Geometry check sheet. Reference: the model listing, model coordinates, mm. A direction names the side the tool comes from. Coordinates: 2 decimals unless noted, no trailing zeros. One line per question, with ' | ' between items.
from build123d import *

# Parameters (mm, degrees)
SKETCH2_W                   = 25.4
SKETCH2_H                   = 25.4
FILLET1_R                   = 3.175
SHELL1_T                    = -1.5875
SKETCH3_R                   = 3.175
WOOD_HOLE_DEPTH             = 1.5875
LPATTERN1_COUNT             = 7
LPATTERN1_PITCH             = 63.5
SKETCH5_R                   = 3.175
CONT_MTG_DEPTH              = 470.9
F_1_4_0_25_DIAMETER_HOLE1_D = 6.35
SKETCH8_R                   = 3.571875
CUT_EXTRUDE1_DEPTH          = 26.4
LPATTERN2_COUNT             = 2
LPATTERN2_PITCH             = 25.4


with BuildPart() as part:
    # Base-Sweep: sweep along a path in Sketch1
    with BuildLine(Plane.XY) as base_sweep_path:
        Line((0, 0), (406.4, 0))
        ThreePointArc((406.4, 0), (442.321024484, -14.878975516), (457.2, -50.8))
        Line((457.2, -50.8), (457.2, -914.4))
    # Sketch2 (on Right Plane) → Base-Sweep (sweep)
    with BuildSketch(Plane(origin=(0, 0, 0), x_dir=(0, 0, -1), z_dir=(1, 0, 0))):
        Rectangle(SKETCH2_W, SKETCH2_H)
    sweep(path=base_sweep_path.line)

    # Fillet1
    fillet1_edges = [part.edges().sort_by_distance(p)[0] for p in [
        (451.301280605, -5.898719395, 12.7),
        (451.301280605, -5.898719395, -12.7),
        (433.340768363, -23.859231637, -12.7),
        (433.340768363, -23.859231637, 12.7),
        (469.9, -482.6, 12.7),
        (469.9, -482.6, -12.7),
        (444.5, -482.6, -12.7),
        (444.5, -482.6, 12.7),
        (203.2, 12.7, 12.7),
        (203.2, 12.7, -12.7),
        (203.2, -12.7, -12.7),
        (203.2, -12.7, 12.7),
    ]]
    fillet(fillet1_edges, radius=FILLET1_R)

    # Shell1
    shell1_openings = [part.faces().sort_by_distance(p)[0] for p in [
        (457.2, -914.4, 0),
        (0, 0, 0),
    ]]
    offset(amount=SHELL1_T, openings=shell1_openings, kind=Kind.INTERSECTION)

    # Sketch3 → Wood Hole (cut)
    with BuildSketch(Plane(origin=(0, 12.7, 0), x_dir=(-1, 0, 0), z_dir=(0, 1, 0))):
        with Locations((-12.7, 0)):
            Circle(SKETCH3_R)
    wood_hole = extrude(amount=-WOOD_HOLE_DEPTH, mode=Mode.SUBTRACT)

    # LPattern1: Wood Hole ×7
    with Locations(*[(i * LPATTERN1_PITCH, 0, 0) for i in range(1, LPATTERN1_COUNT)]):
        add(wood_hole, mode=Mode.SUBTRACT)

    # Sketch5 → cont_mtg (cut, through all)
    with BuildSketch(Plane(origin=(469.9, 0, 0), x_dir=(0, 0, -1), z_dir=(1, 0, 0))):
        with Locations((0, -109.5375)):
            Circle(SKETCH5_R)
        with Locations((0, -134.9375)):
            Circle(SKETCH5_R)
    extrude(amount=-CONT_MTG_DEPTH, mode=Mode.SUBTRACT)

    # 1/4 (0.25) Diameter Hole1 (through all)
    with Locations(Plane.XY.offset(12.7)):
        with Locations((177.8, 0), (355.6, 0)):
            Hole(F_1_4_0_25_DIAMETER_HOLE1_D / 2)

    # Sketch8 → Cut-Extrude1 (cut, through all)
    with BuildSketch(Plane(origin=(0, 0, -12.7), x_dir=(-1, 0, 0), z_dir=(0, 0, -1))):
        with Locations((-457.2, -889)):
            Circle(SKETCH8_R)
    cut_extrude1 = extrude(amount=-CUT_EXTRUDE1_DEPTH, mode=Mode.SUBTRACT)

    # LPattern2: Cut-Extrude1 ×2
    with Locations(*[(0, i * LPATTERN2_PITCH, 0) for i in range(1, LPATTERN2_COUNT)]):
        add(cut_extrude1, mode=Mode.SUBTRACT)


solid = part.part
1. Go/stop test with flat-tipped pins: P1, Ø10, axis at y = -134.94, z = 0, coming from the -X side; P2, Ø10, axis at x = 139.7, z = 0, coming from the -Y side; P3, Ø5, axis at x = 12.7, z = 0, coming from the +Y side; P4, Ø7.5, axis at x = 177.8, y = 0, coming from the -Z side. Record where each tip stops, or that it passes through.
Worked answers:
P1: x = 444.5 | P2: y = -12.7 | P3: y = -11.11 | P4: z = -12.7
2. Material ranges on line 1 (Y direction, x = 175, z = -8); line 2 (X direction, y = -116, z = -0.25); line 3 (Y direction, x = 177.8, z = -12.2) (3 decimals), recorded low to high. Write a range as from..to.
Worked answers:
line 1: -12.7..-11.11, 11.11..12.7 | line 2: 444.5..446.09, 468.31..469.9 | line 3: -11.235..-3.175, 3.175..11.235
3. Tool access check on faces 5 (the face through (206, -11.112, 0)), 6 (the face through (468.312, -489, 0)), 7 (the face through (434.153, -22.43, -0.133)), 8 (the face through (206, -12.7, 0)), 9 (the face through (0, -1, -11.3)). Record the directions out of +Z, -Z, +X, -X, +Y, -Y that give a thin tool (end or side, any length) a straight path to the whole face; none if there is none.
Worked answers:
face 5: -X | face 6: -Y | face 7: none | face 8: +Z, -Z, -X, -Y | face 9: +Z, -Z, -X, +Y, -Y
4. Mould release check, pull along X, two halves, no side actions. Record for faces 1 (the face through (206, 11.112, 2)), 2 (the face through (444.5, -489, 0)), 3 (the face through (449.69, -6.54, 0.13)), 4 (the face through (450.805, -5.408, 0.133)): released by +X, released by -X, zero draft, split by the parting line, or undercut.
Worked answers:
face 1: zero draft | face 2: released by -X | face 3: undercut | face 4: released by +X
